Could you check a few things on this drawing? It's one solid part, dimensions in mm from its lowest x, y, z. A direction names the side the tool comes from. Give positions to 0.01 mm unless a question says otherwise; leave off trailing zeros. Loops run counter-clockwise (first coordinate to the right, second up) from the corner with the lowest first, then second, coordinate; pieces in that order, holes last. Notation, with made-up numbers: M 42,-28.5 L 81,-28.5 A11 ccw 81,-8.5 Z; hole C 31.25,-33.5 d6. An arc over 180 degrees is marked long. Answer as a JSON object with one key per item and string values.
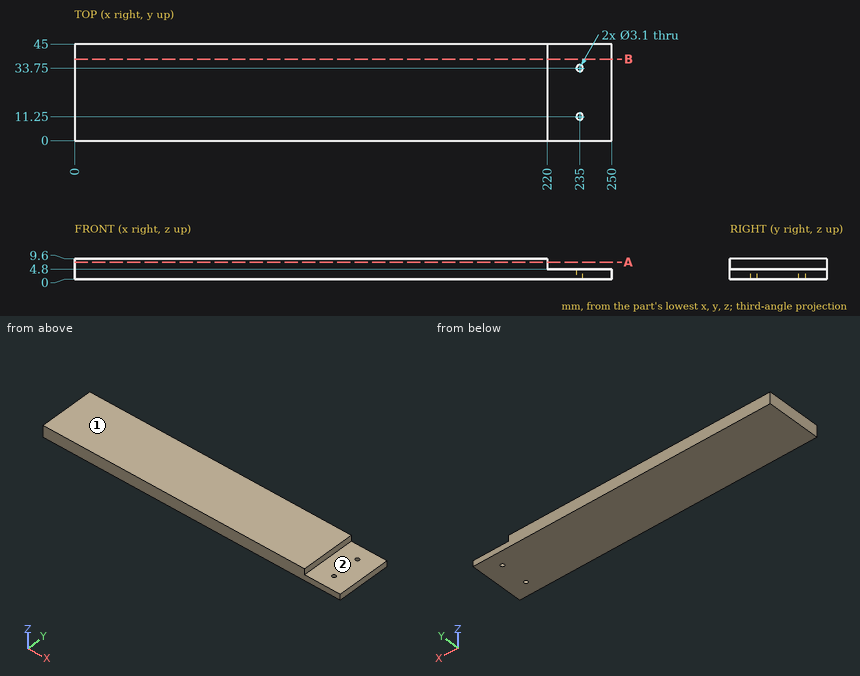
1) Please list where these lines run through material, in increasing order: line 1 along Y through (x, z) = (235, 2.2); line 2 along X through (y, z) = (11.25, 3.4); line 3 along X through (y, z) = (26, 5.25). Write a range as from..to.
Answer list:
{"line 1": "0..9.7, 12.8..32.2, 35.3..45", "line 2": "0..233.45, 236.55..250", "line 3": "0..220"}
2) For the marked faces 1 and 2, which set-ups out of +Z, -Z, +X, -X, +Y, -Y let a thin tool reach every point of the face, with its end or its side?
Answer list:
{"face 1": "+Z, +X, -X, +Y, -Y", "face 2": "+Z, +X, +Y, -Y"}
3) Will this pin go through, and if not, where does the flat tip stop? pin 1 Ø4 at (y, z) = (22, 8) entering from +X.
Answer list:
{"pin 1": "x = 220"}
4) Suppose I cut it at B-B, the plane y = 38. Write out the boundary of the cut face in (x, z), and give its area (3 significant figures).
Answer list:
{"outline": "M 0,0 L 250,0 L 250,4.8 L 220,4.8 L 220,9.6 L 0,9.6 Z", "area": "2,260 mm^2"}
5) Suppose I cut it at A-A, the plane z = 8. Write out the boundary of the cut face in (x, y).
Answer list:
{"outline": "M 0,0 L 220,0 L 220,45 L 0,45 Z"}
